```python
from build123d import *

# Parameters (mm, degrees)
F4_W     = 390
F4_H     = 250
F5_DEPTH = 280
F6_SIZE2 = 149.99999
F6_SIZE  = 279.99999
F7_T     = 8


# Not quite as in the source:
# - a fillet or chamfer is up to 0.001 mm smaller than in the source, because OpenCascade refuses the exact size
# - a shell that OpenCascade refuses in one call is made with other operations: the cavity is built on its own and cut out


with BuildPart() as f5:
    # F4 (on Top) → F5 (new body)
    with BuildSketch(Plane.XY):
        with Locations((9.861856699, -53.0331014672)):
            Rectangle(F4_W, F4_H)
    extrude(amount=F5_DEPTH)

    # F6 (size 280 and 150 in the source; OpenCascade refuses exactly that, so slightly less here)
    f6_edges = [f5.edges().sort_by_distance(p)[0] for p in [
        (9.861857, 71.966899, 280),
    ]]
    f6_side = f5.faces().sort_by_distance((9.861857, 71.966899, 140))[0]
    chamfer(f6_edges, length=F6_SIZE, length2=F6_SIZE2, reference=f6_side)

    # F7: shell of thickness 8, made by hand


with BuildPart() as f7_core1:
    # F7_t2: copy of F5
    add(f5.part)

    # the walls: a layer under each face that stays
    f7_faces = [f7_core1.faces().sort_by_distance(p)[0] for p in [
        (-185.138143301, -53.0331014672, 140),
        (9.861856699, 71.9668985328, 5e-06),
        (9.861856699, -3.0330964672, 140.000005),
        (9.861856699, -128.0330964672, 280),
        (9.861856699, -178.0331014672, 140),
        (204.861856699, -53.0331014672, 140),
    ]]
    thicken(f7_faces, amount=-F7_T, mode=Mode.SUBTRACT)


with BuildPart() as f5_1:
    add(f5.part)

    # what is left inside the walls is the cavity
    f7_cavity = [f7_core1.part.solids().sort_by_distance(p)[0] for p in [
        (9.861857, 14.249313, 90.628889),
    ]]
    add(f7_cavity, mode=Mode.SUBTRACT)


solid = f5_1.part
```
Geometry: final body of the model. Coordinates: model frame, mm. A direction names the side the tool comes from. Give positions to 0.01 mm unless a question says otherwise; leave off trailing zeros. Write each loop counter-clockwise with the first axis right and the second up, starting at its lowest first coordinate (ties: lowest second). Pieces come first, ordered by that corner, then holes.
1. Line query: probe 1 along X at (y, z) = (-53, 157); probe 2 along Y at (x, z) = (-27.5, 114); probe 3 along Y at (x, z) = (0, 51.5). Output: solid intervals per line, ascending.
2. Draft query along Y for faces 1 (the flat face through (7, -127, 280)), 2 (the flat face through (-177.138, -81, 104)), 3 (the flat face through (7, -126, 272)), 4 (the flat face through (7, -178.033, 138)). Return one class per face: released by +Y, released by -Y, zero draft, split by the parting line, or undercut.
3. Section query C-C, the plane y = 32. Return loops of the section in (x, z).
4. Pin query (flat end, axial travel): P1, Ø12, axis at x = -127.5, y = -95, coming from the -Z side; P2, Ø1, axis at x = 109, z = 144.5, coming from the +Y side; P3, Ø4, axis at x = 76.5, z = 198, coming from the +Y side. Return the tip coordinate at first contact, or that it passes through.
5. Section query D-D, the plane z = 206. Return loops of the section in (x, y).
6. Reachability of faces 5 (the flat face through (7.244, -10.986, 137.904)), 6 (the flat face through (204.862, -83, 107)) from +Z, -Z, +X, -X, +Y, -Y: full face, straight path, thin tool, end or side. Return the list, or none.
7. Section query B-B, the plane z = 38.5. Return loops of the section in (x, y).
Computed:
1. probe 1: x = -185.14 to -177.14, 196.86 to 204.86
1. probe 2: y = -178.03 to -170.03, 1.82 to 10.9
1. probe 3: y = -178.03 to -170.03, 35.3 to 44.38
2. face 1: zero draft
2. face 2: undercut
2. face 3: undercut
2. face 4: released by -Y
3. outline: (-185.14, 0) - (-177.14, 0) - (-177.14, 57.66) - (196.86, 57.66) - (196.86, 0) - (204.86, 0) - (204.86, 74.6) - (-185.14, 74.6) - close
4. P1: stops at z = 272
4. P2: stops at y = -5.18
4. P3: stops at y = -33.03
5. outline: (-185.14, -178.03) - (204.86, -178.03) - (204.86, -38.39) - (-185.14, -38.39) - close; hole (-177.14, -170.03) - (196.86, -170.03) - (196.86, -47.47) - (-177.14, -47.47) - close
6. face 5: -Z
6. face 6: +Z, -Z, +X, +Y, -Y
7. outline: (-185.14, -178.03) - (204.86, -178.03) - (204.86, 51.34) - (-185.14, 51.34) - close; hole (-177.14, -170.03) - (196.86, -170.03) - (196.86, 42.27) - (-177.14, 42.27) - close
